Design review of the part shown in the three views and the two pictorial views. Dimensions are in mm from the part's minimum x, y and z. A direction names the side the tool comes from. Give positions to 0.01 mm unless a question says otherwise; leave off trailing zeros. Write each loop counter-clockwise with the first axis right and the second up, starting at its lowest first coordinate (ties: lowest second). Pieces come first, ordered by that corner, then holes. Notation, with made-up numbers: (-8, 78) -> (50, 78) arc R14 cw to (50, 104) -> close; hole circle Ø11 at (50, 54.5). An arc over 180 degrees is marked (long way). Return JSON: item names as keys, results as strings. Group by question number.
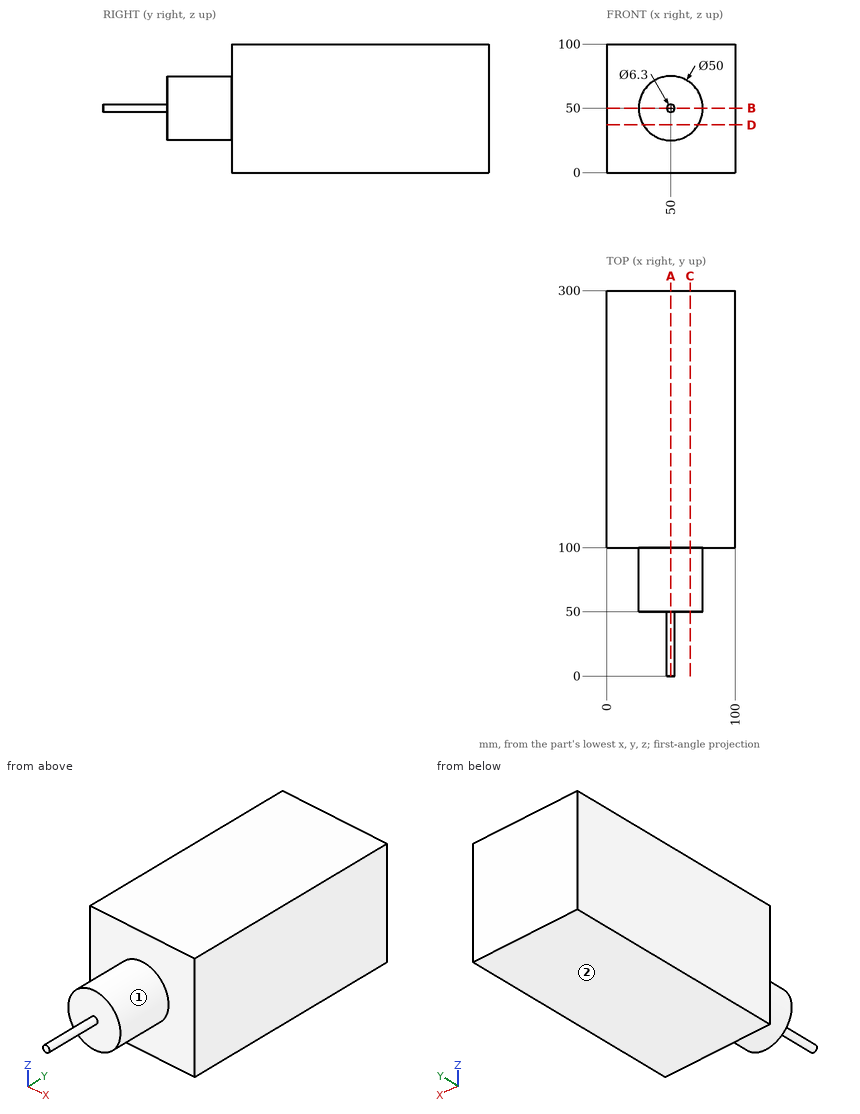
Q1. Tool access review of the marked faces 1 and 2: name each direction out of +Z, -Z, +X, -X, +Y, -Y from which nothing blocks a thin tool from reaching the whole face with its end or side.
Q2. Take a section at C-C, the plane x = 65. Give the boundary of the cut face in (y, z), plus the area to 3 significant figures.
Q3. Take a section at A-A, the plane x = 50. Give the boundary of the cut face in (y, z).
Q4. For L1, parallel to Y at x = 80.5, z = 15.5, list the stretches that pass through material, from the lowest coordinate up. Write a range as from..to.
Q5. Insertion check: pin 1 (4 mm diameter, centred on x = 38, y = 215, fed in from -Z); pin 2 (6 mm diameter, centred on x = 58, z = 36, fed in from -Y); pin 3 (1.5 mm diameter, centred on x = 12.5, z = 23, fed in from -Y). Each pin has a flat end and moves straight along its axis. Give the tip position at first contact, or say it passes through.
Q6. Take a section at B-B, the plane z = 50. Give the boundary of the cut face in (x, y).
Q7. Take a section at D-D, the plane z = 37. Give the boundary of the cut face in (x, y), plus the area to 3 significant figures.
Final values:
{
 "1": {"face 1": "-Y", "face 2": "-Z, +X, -X, +Y, -Y"},
 "2": {"outline": "(50, 30) -> (100, 30) -> (100, 0) -> (300, 0) -> (300, 100) -> (100, 100) -> (100, 70) -> (50, 70) -> close", "area": "22,000 mm²"},
 "3": {"outline": "(0, 46.85) -> (50, 46.85) -> (50, 25) -> (100, 25) -> (100, 0) -> (300, 0) -> (300, 100) -> (100, 100) -> (100, 75) -> (50, 75) -> (50, 53.15) -> (0, 53.15) -> close"},
 "4": {"L1": "y = 100..300"},
 "5": {"pin 1": "stops at z = 0", "pin 2": "stops at y = 50", "pin 3": "stops at y = 100"},
 "6": {"outline": "(0, 100) -> (25, 100) -> (25, 50) -> (46.85, 50) -> (46.85, 0) -> (53.15, 0) -> (53.15, 50) -> (75, 50) -> (75, 100) -> (100, 100) -> (100, 300) -> (0, 300) -> close"},
 "7": {"outline": "(0, 100) -> (28.65, 100) -> (28.65, 50) -> (71.35, 50) -> (71.35, 100) -> (100, 100) -> (100, 300) -> (0, 300) -> close", "area": "22,100 mm²"}
}
